Geometry: final body of the model. Coordinates: model frame, mm. Coordinates: 2 decimals unless noted, no trailing zeros. Write each loop counter-clockwise with the first axis right and the second up, starting at its lowest first coordinate (ties: lowest second). Pieces come first, ordered by that corner, then holes. Notation, with made-up numbers: (71.25, 72.5) - (102.25, 72.5) arc R27 cw to (102.25, 96.5) - close; hole circle Ø7 at (-22.75, 23.25). An arc over 180 degrees is marked (long way). Put each result on its own line as item: value.
```python
from build123d import *

# Parameters (mm, degrees)
F0_W     = 80
F0_H     = 80
F1_DEPTH = 80
F2_R     = 16.82409
F3_DEPTH = 80.001
F4_R     = 5


with BuildPart() as f1:
    # F0 (on Top) → F1 (new body)
    with BuildSketch(Plane.XY):
        with Locations((-54.952934, 27.584402)):
            Rectangle(F0_W, F0_H)
    extrude(amount=F1_DEPTH)

    # F2 (on face) → F3 (cut, through all)
    with BuildSketch(Plane.XY.offset(80)):
        with Locations((-55.576466, 27.750002)):
            Circle(F2_R)
    extrude(amount=-F3_DEPTH, mode=Mode.SUBTRACT)

    # F4
    f4_edges = [f1.edges().sort_by_distance(p)[0] for p in [
        (-54.952934, 67.584402, 80),
        (-94.952934, 27.584402, 80),
        (-54.952934, -12.415598, 80),
        (-14.952934, 27.584402, 80),
    ]]
    fillet(f4_edges, radius=F4_R)


solid = f1.part
```
1. Ray query, probe 1 along X at (y, z) = (27, 24); probe 2 along X at (y, z) = (29.5, 55.5); probe 3 along Y at (x, z) = (-63.5, 43.5). Return the intervals inside material, ascending. Write a range as from..to.
Answer below:
probe 1: x = -94.95..-72.38, -38.77..-14.95
probe 2: x = -94.95..-72.31, -38.84..-14.95
probe 3: y = -12.42..12.91, 42.59..67.58
2. Section query A-A (x = -43.5). Return loops of the section in (y, z), then the cut area to 3 significant figures.
Answer below:
outline: (-12.42, 0) - (16.04, 0) - (16.04, 80) - (-7.42, 80) arc R5 ccw to (-12.42, 75) - close; (39.46, 0) - (67.58, 0) - (67.58, 75) arc R5 ccw to (62.58, 80) - (39.46, 80) - close
area: 4,520 mm²
3. Section query B-B (y = 31). Return loops of the section in (x, z), then the cut area to 3 significant figures.
Answer below:
outline: (-94.95, 0) - (-72.08, 0) - (-72.08, 80) - (-89.95, 80) arc R5 ccw to (-94.95, 75) - close; (-39.07, 0) - (-14.95, 0) - (-14.95, 75) arc R5 ccw to (-19.95, 80) - (-39.07, 80) - close
area: 3,750 mm²
4. Mould query, pull axis Y, two halves, no side actions, for faces 1 (the flat face through (-38, 28, 0)), 2 (the cylindrical face through (-57.77, 44.43, 40.56)), 3 (the cylindrical face through (-54.393, 66.159, 78.496)). Classes: +Y half, -Y half, draft (parallel to the pull), parting line (faces both ways), or undercut.
Answer below:
face 1: draft
face 2: undercut
face 3: +Y half
5. Section query C-C (z = 52). Return loops of the section in (x, y), then the cut area to 3 significant figures.
Answer below:
outline: (-94.95, -12.42) - (-14.95, -12.42) - (-14.95, 67.58) - (-94.95, 67.58) - close; hole circle Ø33.65 at (-55.58, 27.75)
area: 5,510 mm²
